Source: three-view drawing plus pictorial views. Frame: mm from the lowest corner of the part. Give positions to 0.01 mm unless a question says otherwise; leave off trailing zeros. Loops run counter-clockwise (first coordinate to the right, second up) from the corner with the lowest first, then second, coordinate; pieces in that order, holes last. Notation, with made-up numbers: (-23, 25) - (9, 25) arc R28 ccw to (9, 50) - close; hole circle Ø3 at (-17.5, -14.75). An arc over 180 degrees is marked (long way). Answer in a Markdown table with one row per item.
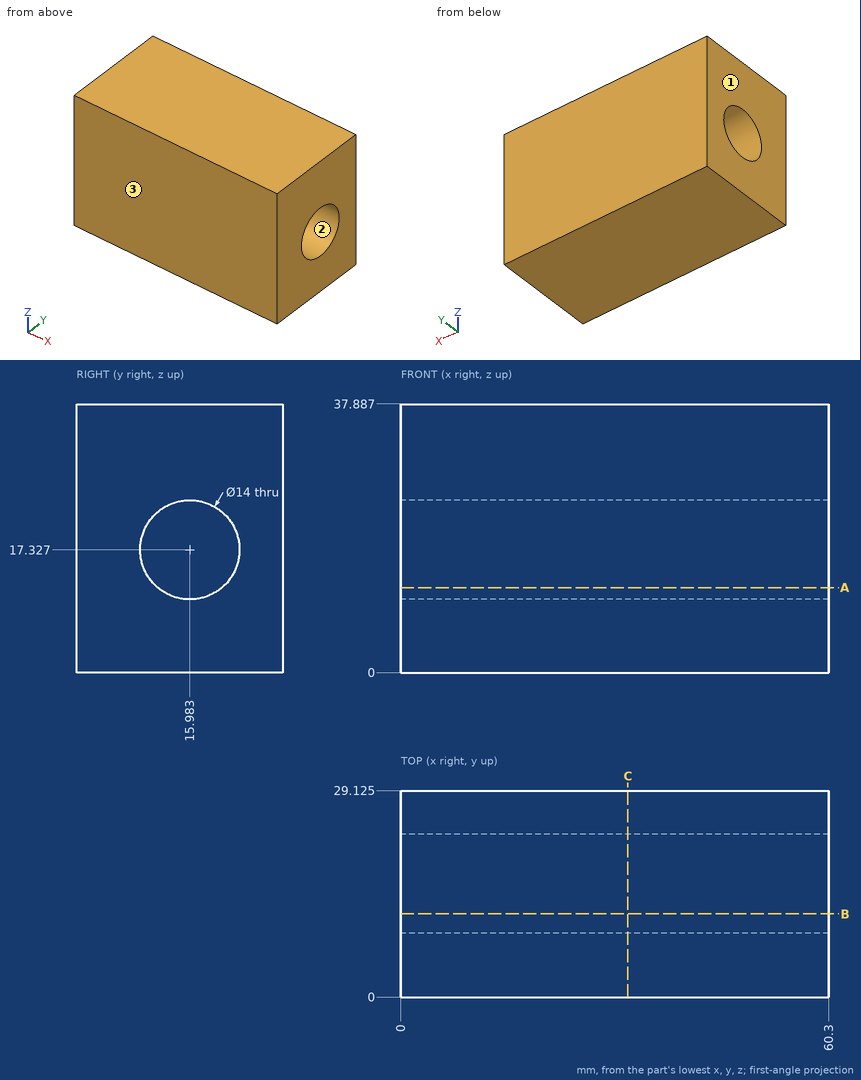
Q1. Material intervals for line 1 along Y through (x, z) = (48, 12) (1 decimal); line 2 along Y through (x, z) = (17, 14.5) (1 decimal); line 3 along Z through (x, y) = (30, 9.75) (1 decimal), sorted ascending.
Check values:
| item | result |
|---|---|
| line 1 | 0 to 11.4, 20.5 to 29.1 |
| line 2 | 0 to 9.6, 22.4 to 29.1 |
| line 3 | 0 to 14.1, 20.5 to 37.9 |
Q2. Cut plane C-C (x = 32). Output: boundary loops of the cut face in (y, z) (1 decimal).
Check values:
| item | result |
|---|---|
| outline | (0, 0) - (29.1, 0) - (29.1, 37.9) - (0, 37.9) - close; hole circle Ø14 at (16, 17.3) |
Q3. First-contact query: pin 1 (4 mm diameter, centred on y = 4, z = 28, fed in from -X). Flat tip, straight axial feed; report the tip coordinate or a pass-through.
Check values:
| item | result |
|---|---|
| pin 1 | x = 0 |
Q4. Cut plane A-A (z = 12). Output: boundary loops of the cut face in (x, y) (1 decimal).
Check values:
| item | result |
|---|---|
| outline | (0, 0) - (60.3, 0) - (60.3, 11.4) - (0, 11.4) - close; (0, 20.5) - (60.3, 20.5) - (60.3, 29.1) - (0, 29.1) - close |
Q5. Draft query along Y for the marked faces 1, 2 and 3. Return one class per face: pulls with the +Y half, pulls with the -Y half, needs draft (parallel to the pull), parting line crosses it, or undercut.
Check values:
| item | result |
|---|---|
| face 1 | needs draft |
| face 2 | undercut |
| face 3 | pulls with the -Y half |
Q6. Cut plane B-B (y = 11.75). Output: boundary loops of the cut face in (x, z).
Check values:
| item | result |
|---|---|
| outline | (0, 0) - (60.3, 0) - (60.3, 11.75) - (0, 11.75) - close; (0, 22.9) - (60.3, 22.9) - (60.3, 37.89) - (0, 37.89) - close |
